Source: CAD feature listing. Evaluate the final solid. Frame: model axes, mm. Face numbers are marked on the shaded views. Give positions to 0.01 mm unless a question says otherwise; leave off trailing zeros. Write each loop counter-clockwise with the first axis right and the second up, starting at its lowest first coordinate (ties: lowest second). Pieces come first, ordered by that corner, then holes. Notation, with made-up numbers: (28, 32) -> (85, 32) arc R17 ccw to (85, 63) -> close; hole circle Ø9 at (44.25, 5.25). An arc over 180 degrees is marked (long way). Write item = value, one per line.
from build123d import *

# Parameters (mm, degrees)
SKETCH1_W           = 30
SKETCH1_H           = 80
SKETCH1_R           = 10
BOSS_EXTRUDE1_DEPTH = 5
SKETCH2_W           = 10
SKETCH2_H           = 10
SKETCH2_R           = 3.25
BOSS_EXTRUDE2_DEPTH = 10


with BuildPart() as part:
    # Sketch1 → Boss-Extrude1 (new body, symmetric)
    with BuildSketch(Plane.XY):
        Rectangle(SKETCH1_W, SKETCH1_H)
        with Locations((0, 28)):
            Circle(SKETCH1_R, mode=Mode.SUBTRACT)
    extrude(amount=BOSS_EXTRUDE1_DEPTH, both=True)

    # Sketch2 → Boss-Extrude2 (add)
    with BuildSketch(Plane.XZ.offset(40)):
        with Locations((20, 0)):
            Rectangle(SKETCH2_W, SKETCH2_H)
        with Locations((20, 0)):
            Circle(SKETCH2_R, mode=Mode.SUBTRACT)
    boss_extrude2 = extrude(amount=-BOSS_EXTRUDE2_DEPTH)

    # Mirror1: Boss-Extrude2 across plane
    add(boss_extrude2.mirror(Plane(origin=(0, 0, 0), x_dir=(0, 0, 1), z_dir=(1, 0, 0))))


solid = part.part
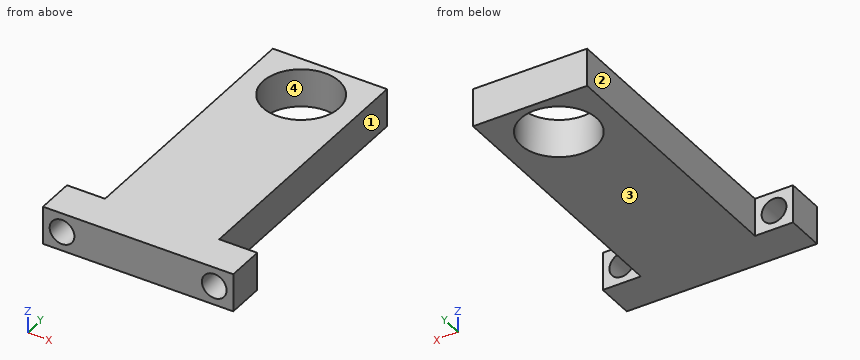
(1) Section query B-B (x = 5). Return loops of the section in (y, z).
Values follow:
outline = (-40, -5) -> (19.34, -5) -> (19.34, 5) -> (-40, 5) -> close; (36.66, -5) -> (40, -5) -> (40, 5) -> (36.66, 5) -> close
(2) Section query D-D (y = -31). Return loops of the section in (x, z).
Values follow:
outline = (-25, -5) -> (25, -5) -> (25, 5) -> (-25, 5) -> close; hole circle Ø6.5 at (-20, 0); hole circle Ø6.5 at (20, 0)
(3) Section query A-A (z = 0). Return loops of the section in (x, y).
Values follow:
outline = (-25, -40) -> (-23.25, -40) -> (-23.25, -30) -> (-25, -30) -> close; (-16.75, -40) -> (16.75, -40) -> (16.75, -30) -> (15, -30) -> (15, 40) -> (-15, 40) -> (-15, -30) -> (-16.75, -30) -> close; (23.25, -40) -> (25, -40) -> (25, -30) -> (23.25, -30) -> close; hole circle Ø20 at (0, 28)
(4) Section query C-C (y = 22.5). Return loops of the section in (x, z), plus the area to 3 significant figures.
Values follow:
outline = (-15, -5) -> (-8.35, -5) -> (-8.35, 5) -> (-15, 5) -> close; (8.35, -5) -> (15, -5) -> (15, 5) -> (8.35, 5) -> close
area = 133 mm2
(5) Pull-direction query (X, two-part tool) for the marked faces 1, 2, 3 and 4; classes: pulls with the +X half, pulls with the -X half, needs draft (parallel to the pull), parting line crosses it, or undercut.
Values follow:
face_1 = pulls with the +X half
face_2 = pulls with the -X half
face_3 = needs draft
face_4 = undercut
(6) First-contact query: pin 1 (12 mm diameter, centred on x = 0, y = 28, fed in from +Z); pin 2 (2 mm diameter, centred on y = 23.5, z = 1.5, fed in from -X); pin 3 (1.5 mm diameter, centred on x = -16, z = 3.5, fed in from +Y); pin 4 (1 mm diameter, centred on y = -14.5, z = -3.5, fed in from +X). Flat tips, straight axial feed; report the tip coordinate or a pass-through.
Values follow:
pin_1 = through
pin_2 = -15
pin_3 = -30
pin_4 = 15
(7) Material intervals for line 1 (Z direction, x = -20, y = -32.5); line 2 (X direction, y = 4, z = -1.75); line 3 (Y direction, x = -2.5, z = -2), sorted ascending.
Values follow:
line_1 = -5 to -3.25, 3.25 to 5
line_2 = -15 to 15
line_3 = -40 to 18.32, 37.68 to 40
